from build123d import *


with BuildPart() as part:
    # Sketch3 → Revolve3 (revolve)
    with BuildSketch(Plane(origin=(0, 0, 0), x_dir=(0, 0, -1), z_dir=(1, 0, 0))):
        with BuildLine():
            ThreePointArc((7.976750754, 22.176677088), (11.759040062, 36.040371448), (0, 44.300680797))
            Line((0, 44.300680797), (0, 22.176677088))
            Line((0, 22.176677088), (0, 20.176677088))
            Line((0, 20.176677088), (0, 19.300680797))
            Line((0, 19.300680797), (0, -18.199319203))
            Line((0, -18.199319203), (0, -30.699319203))
            Line((0, -30.699319203), (17.300215532, -30.699319203))
            Line((17.300215532, -30.699319203), (20, -30.699319203))
            Line((20, -30.699319203), (19.055215287, -18.889510286))
            ThreePointArc((19.055215287, -18.889510286), (18.816349006, -18.398249022), (18.307603828, -18.199319203))
            Line((18.307603828, -18.199319203), (17, -18.199319203))
            Line((17, -18.199319203), (15.404164559, -8.225347699))
            ThreePointArc((15.404164559, -8.225347699), (14.556848822, -6.571703413), (12.898197127, -5.734232256))
            Line((12.898197127, -5.734232256), (8.329404716, 20.176677088))
            Line((8.329404716, 20.176677088), (11.25, 20.176677088))
            ThreePointArc((11.25, 20.176677088), (11.780330086, 20.396347002), (12, 20.926677088))
            Line((12, 20.926677088), (12, 21.426677088))
            ThreePointArc((12, 21.426677088), (11.780330086, 21.957007173), (11.25, 22.176677088))
            Line((11.25, 22.176677088), (7.976750754, 22.176677088))
        make_face()
    revolve(axis=Axis((0, 63.905153842, 0), (0, -1, 0)))


solid = part.part
Could you check a few things on this model? Use its own coordinates, in mm. A direction names the side the tool comes from. Give positions to 0.01 mm unless a question says otherwise; leave off trailing zeros. Order: outer loops, then holes, each group sorted by start corner. A loop starts at its lowest first (then second) coordinate and runs counter-clockwise, first axis right, second up.
1. I need wall thicknesses on L1, parallel to Y at x = 3, z = 18; L2, parallel to Z at x = -7, y = -24; L3, parallel to Z at x = -8, y = 18. Which ranges of each line are inside material? Lowest first, please.
Answers below:
L1: y = -30.7 to -18.2
L2: z = -18.16 to 18.16
L3: z = -3.45 to 3.45
2. Which directions (+Z, -Z, +X, -X, +Y, -Y) give clear straight access to the entire face, cutting with the end or side of a thin tool? Please do faces 1 (the flat face through (-4, 20.177, -8)), 2 (the flat face through (-13.5, -18.199, -10.8)).
Answers below:
face 1: none
face 2: +Y
3. Thinking about a two-plate mould opening in Y: for faces 3 (the flat face through (-2, 22.177, 8)), 4 (the conical face through (-15.46, -10.93, 3.43)), 5 (the conical face through (3.03, 10.28, -9.61)), 6 (the flat face through (0, -30.699, 0)), which applies, +Y half, -Y half, draft (parallel to the pull), parting line (faces both ways), or undercut?
Answers below:
face 3: undercut
face 4: +Y half
face 5: undercut
face 6: -Y half
4. For pin 1 (8 mm diameter, centred on y = -18.5, z = -15.5, fed in from +X); pin 2 (5 mm diameter, centred on x = -3, z = -10.5, fed in from +Y); pin 3 (1 mm diameter, centred on x = 7, z = 0, fed in from +Y); pin 4 (6 mm diameter, centred on y = 14.5, z = -15, fed in from +X), each with a flat end and sliding along its axis, tell me the tip position at first contact or that it passes through.
Answers below:
pin 1: stops at x = 15.18
pin 2: stops at y = 41.04
pin 3: stops at y = 42.48
pin 4: passes through
5. Suppose I cut it at B-B (x = 0). Write out the boundary of the cut face in (y, z), plus the area to 3 significant figures.
Answers below:
outline: (-30.7, -20) - (-18.89, -19.06) arc R0.75 ccw to (-18.2, -18.31) - (-18.2, -17) - (-8.23, -15.4) arc R3 ccw to (-5.73, -12.9) - (20.18, -8.33) - (20.18, -11.25) arc R0.75 ccw to (20.93, -12) - (21.43, -12) arc R0.75 ccw to (22.18, -11.25) - (22.18, -7.98) arc R12.5 ccw (long way) to (22.18, 7.98) - (22.18, 11.25) arc R0.75 ccw to (21.43, 12) - (20.93, 12) arc R0.75 ccw to (20.18, 11.25) - (20.18, 8.33) - (-5.73, 12.9) arc R3 ccw to (-8.23, 15.4) - (-18.2, 17) - (-18.2, 18.31) arc R0.75 ccw to (-18.89, 19.06) - (-30.7, 20) - close
area: 1,940 mm2
6. Suppose I cut it at C-C (z = -9.5). State how many separate pieces and enclosed holes the cut face has, plus the area to 3 significant figures.
Answers below:
separate pieces: 3
enclosed holes: 0
area: 1,200 mm2
7. Suppose I cut it at A-A (z = 0). Write out the boundary of the cut face in (x, y).
Answers below:
outline: (-20, -30.7) - (20, -30.7) - (19.06, -18.89) arc R0.75 ccw to (18.31, -18.2) - (17, -18.2) - (15.4, -8.23) arc R3 ccw to (12.9, -5.73) - (8.33, 20.18) - (11.25, 20.18) arc R0.75 ccw to (12, 20.93) - (12, 21.43) arc R0.75 ccw to (11.25, 22.18) - (7.98, 22.18) arc R12.5 ccw (long way) to (-7.98, 22.18) - (-11.25, 22.18) arc R0.75 ccw to (-12, 21.43) - (-12, 20.93) arc R0.75 ccw to (-11.25, 20.18) - (-8.33, 20.18) - (-12.9, -5.73) arc R3 ccw to (-15.4, -8.23) - (-17, -18.2) - (-18.31, -18.2) arc R0.75 ccw to (-19.06, -18.89) - close
8. Suppose I cut it at D-D (y = 30.5). Write out the boundary of the cut face in (x, z), plus the area to 3 significant figures.
Answers below:
outline: circle Ø24.86 at (0, 0)
area: 486 mm2
